Source: CAD feature listing. Evaluate the final solid. Frame: model axes, mm. A direction names the side the tool comes from. Give positions to 0.01 mm unless a question says otherwise; leave off trailing zeros. Order: outer loops, then holes, each group sorted by start corner. A loop starts at its lowest first (then second) coordinate and runs counter-clockwise, first axis right, second up.
from build123d import *

# Parameters (mm, degrees)
SKETCH_1_W           = 15
SKETCH_1_H           = 3
EXTRUDE_1_DEPTH      = 3
SKETCH_2_W           = 15
SKETCH_2_H           = 3
EXTRUDE_2_DEPTH      = 0.5
FILLET_2_R           = 3
FILLET_3_R           = 0.5
FILLET_4_R           = 0.5
SKETCH_6_W           = 103.474287265
SKETCH_6_H           = 3
CUT_EXTRUDE_3_DEPTH  = 10
FILLET_5_R           = 0.5
FILLET_6_R           = 0.5
SKETCH_15_W          = 15
SKETCH_15_H          = 9
EXTRUDE_4_DEPTH      = 3
FILLET_7_R           = 1
SKETCH_16_R          = 1.5
CUT_EXTRUDE_7_DEPTH  = 188.894654659
SKETCH_17_R          = 1.52921897
SKETCH_17_R_2        = 1.502123086
CUT_EXTRUDE_8_DEPTH  = 188.894654659
EXTRUDE_5_DEPTH      = 3
SKETCH_19_R          = 1.5
CUT_EXTRUDE_9_DEPTH  = 10
EXTRUDE_6_DEPTH      = 3
CUT_EXTRUDE_10_DEPTH = 3


with BuildPart() as part:
    # Sketch 1 → Extrude 1 (new body)
    with BuildSketch(Plane.XY):
        Polygon((0, 101), (0, 0), (157.65, 0), (25, 79), (25, 101), (20, 101), (5, 101), align=None)
        with Locations((12.5, 102.5)):
            Rectangle(SKETCH_1_W, SKETCH_1_H)
    extrude(amount=EXTRUDE_1_DEPTH)

    # Sketch 2 → Extrude 2 (add)
    with BuildSketch(Plane(origin=(0, 104, 0), x_dir=(1, 0, 0), z_dir=(0, 1, 0))):
        with Locations((12.5, -1.5)):
            Rectangle(SKETCH_2_W, SKETCH_2_H)
    extrude(amount=EXTRUDE_2_DEPTH)

    # Fillet 2
    fillet_2_edges = [part.edges().sort_by_distance(p)[0] for p in [
        (25, 79, 1.5),
    ]]
    fillet(fillet_2_edges, radius=FILLET_2_R)

    # Fillet 3
    fillet_3_edges = [part.edges().sort_by_distance(p)[0] for p in [
        (157.65, 0, 1.5),
    ]]
    fillet(fillet_3_edges, radius=FILLET_3_R)

    # Fillet 4
    fillet_4_edges = [part.edges().sort_by_distance(p)[0] for p in [
        (0, 0, 1.5),
    ]]
    fillet(fillet_4_edges, radius=FILLET_4_R)

    # Sketch 6 → Cut-Extrude 3 (cut)
    with BuildSketch(Plane.XY.offset(3)):
        with Locations((71.737143632, 1.5)):
            Rectangle(SKETCH_6_W, SKETCH_6_H)
        with BuildLine():
            Line((5, 3), (0, 3))
            Line((0, 3), (0, 0.5))
            ThreePointArc((0, 0.5), (0.146446609, 0.146446609), (0.5, 0))
            Line((0.5, 0), (5, 0))
            Line((5, 0), (5, 3))
        make_face()
        with BuildLine():
            Line((152.612658228, 3), (138.474287265, 3))
            Line((138.474287265, 3), (138.474287265, 0))
            Line((138.474287265, 0), (155.833275758, 0))
            ThreePointArc((155.833275758, 0), (156.315351251, 0.367322877), (156.089117317, 0.929587124))
            Line((156.089117317, 0.929587124), (152.612658228, 3))
        make_face()
    extrude(amount=-CUT_EXTRUDE_3_DEPTH, mode=Mode.SUBTRACT)

    # Fillet 5
    fillet_5_edges = [part.edges().sort_by_distance(p)[0] for p in [
        (123.474287265, 0, 1.5),
        (20, 0, 1.5),
        (138.474287265, 0, 1.5),
        (152.612658228, 3, 1.5),
        (0, 3, 1.5),
        (5, 0, 1.5),
    ]]
    fillet(fillet_5_edges, radius=FILLET_5_R)

    # Fillet 6
    fillet_6_edges = [part.edges().sort_by_distance(p)[0] for p in [
        (123.474287265, 3, 1.5),
        (20, 3, 1.5),
        (5, 101, 1.5),
        (20, 101, 1.5),
        (138.474287265, 3, 1.5),
        (5, 3, 1.5),
    ]]
    fillet(fillet_6_edges, radius=FILLET_6_R)

    # Sketch 15 → Extrude 4 (add)
    with BuildSketch(Plane(origin=(0, 0, 0), x_dir=(-1, 0, 0), z_dir=(0, 0, -1))):
        with Locations((-12.5, 106.877473525)):
            Rectangle(SKETCH_15_W, SKETCH_15_H)
    extrude(amount=-EXTRUDE_4_DEPTH)

    # Fillet 7
    fillet_7_edges = [part.edges().sort_by_distance(p)[0] for p in [
        (5, 111.377473525, 1.5),
        (20, 111.377473525, 1.5),
    ]]
    fillet(fillet_7_edges, radius=FILLET_7_R)

    # Sketch 16 → Cut-Extrude 7 (cut, through all)
    with BuildSketch(Plane(origin=(0, 0, 0), x_dir=(-1, 0, 0), z_dir=(0, 0, -1))):
        with Locations((-14.568919479, 6)):
            Circle(SKETCH_16_R)
        with Locations((-24.568919479, 6)):
            Circle(SKETCH_16_R)
        with Locations((-123.740220593, 6)):
            Circle(SKETCH_16_R)
        with Locations((-133.740220593, 6)):
            Circle(SKETCH_16_R)
    extrude(amount=-CUT_EXTRUDE_7_DEPTH, mode=Mode.SUBTRACT)

    # Sketch 17 → Cut-Extrude 8 (cut, through all)
    with BuildSketch(Plane.XY.offset(3)):
        with Locations((4.795751321, 98)):
            Circle(SKETCH_17_R)
        with Locations((14.795751321, 98)):
            Circle(SKETCH_17_R_2)
    extrude(amount=-CUT_EXTRUDE_8_DEPTH, mode=Mode.SUBTRACT)

    # Sketch 18 → Extrude 5 (add)
    with BuildSketch(Plane.XY.offset(3)):
        with BuildLine():
            Line((19, 130.377473525), (6, 130.377473525))
            ThreePointArc((6, 130.377473525), (5.292893219, 130.084580306), (5, 129.377473525))
            Line((5, 129.377473525), (5, 110.377473525))
            Line((5, 110.377473525), (20, 110.377473525))
            Line((20, 110.377473525), (20, 129.377473525))
            ThreePointArc((20, 129.377473525), (19.707106781, 130.084580306), (19, 130.377473525))
        make_face()
    extrude(amount=-EXTRUDE_5_DEPTH)

    # Sketch 19 → Cut-Extrude 9 (cut)
    with BuildSketch(Plane.XY.offset(3)):
        with Locations((12.5, 127.377473525)):
            Circle(SKETCH_19_R)
        with Locations((12.5, 118.377473525)):
            Circle(SKETCH_19_R)
    extrude(amount=-CUT_EXTRUDE_9_DEPTH, mode=Mode.SUBTRACT)

    # Sketch 21 → Extrude 6 (add)
    with BuildSketch(Plane.XY.offset(3)):
        with BuildLine():
            Line((25, 101), (151.051775545, 3.929587124))
            Line((151.051775545, 3.929587124), (26.464950647, 78.127545412))
            ThreePointArc((26.464950647, 78.127545412), (25.391825537, 79.222696415), (25, 80.705068154))
            Line((25, 80.705068154), (25, 101))
        make_face()
    extrude(amount=-EXTRUDE_6_DEPTH)

    # Sketch 22 → Cut-Extrude 10 (cut)
    with BuildSketch(Plane(origin=(0, 0, 0), x_dir=(-1, 0, 0), z_dir=(0, 0, -1))):
        with BuildLine():
            Line((-19.9, 19), (-19.9, 87.736313508))
            ThreePointArc((-19.9, 87.736313508), (-16, 91.636313508), (-12.1, 87.736313508))
            Line((-12.1, 87.736313508), (-12.1, 19))
            ThreePointArc((-12.1, 19), (-16, 15.1), (-19.9, 19))
        make_face()
        with BuildLine():
            Line((-26.1, 76.955142244), (-26.1, 19))
            ThreePointArc((-26.1, 19), (-30, 15.1), (-33.9, 19))
            Line((-33.9, 19), (-33.9, 76.955142244))
            ThreePointArc((-33.9, 76.955142244), (-30, 80.855142244), (-26.1, 76.955142244))
        make_face()
        with BuildLine():
            Line((-40.1, 66.17397098), (-40.1, 19))
            ThreePointArc((-40.1, 19), (-44, 15.1), (-47.9, 19))
            Line((-47.9, 19), (-47.9, 66.17397098))
            ThreePointArc((-47.9, 66.17397098), (-44, 70.07397098), (-40.1, 66.17397098))
        make_face()
        with BuildLine():
            Line((-54.1, 55.392799717), (-54.1, 19))
            ThreePointArc((-54.1, 19), (-58, 15.1), (-61.9, 19))
            Line((-61.9, 19), (-61.9, 55.392799717))
            ThreePointArc((-61.9, 55.392799717), (-58, 59.292799717), (-54.1, 55.392799717))
        make_face()
        with BuildLine():
            Line((-68.1, 44.611628453), (-68.1, 19))
            ThreePointArc((-68.1, 19), (-72, 15.1), (-75.9, 19))
            Line((-75.9, 19), (-75.9, 44.611628453))
            ThreePointArc((-75.9, 44.611628453), (-72, 48.511628453), (-68.1, 44.611628453))
        make_face()
        with BuildLine():
            Line((-82.1, 33.830457189), (-82.1, 19))
            ThreePointArc((-82.1, 19), (-86, 15.1), (-89.9, 19))
            Line((-89.9, 19), (-89.9, 33.830457189))
            ThreePointArc((-89.9, 33.830457189), (-86, 37.730457189), (-82.1, 33.830457189))
        make_face()
        with BuildLine():
            Line((-96.1, 23.049285925), (-96.1, 19))
            ThreePointArc((-96.1, 19), (-100, 15.1), (-103.9, 19))
            Line((-103.9, 19), (-103.9, 23.049285925))
            ThreePointArc((-103.9, 23.049285925), (-100, 26.949285925), (-96.1, 23.049285925))
        make_face()
    extrude(amount=-CUT_EXTRUDE_10_DEPTH, mode=Mode.SUBTRACT)


solid = part.part
1) First-contact query: pin 1 Ø0.9 at (y, z) = (43, 2) entering from +X; pin 2 Ø1.5 at (y, z) = (27.5, 1) entering from +X; pin 3 Ø0.6 at (y, z) = (1.5, 1.5) entering from -X. Flat tips, straight axial feed; report the tip coordinate or a pass-through.
Checks:
pin 1: stops at x = 100.9
pin 2: stops at x = 121.42
pin 3: stops at x = 5
2) Ray query, L1, parallel to Y at x = 12.5, z = 1.2; L2, parallel to Y at x = 11.5, z = 0.9; L3, parallel to X at y = 40, z = 0.2. Return the intervals inside material, ascending.
Checks:
L1: y = 0 to 17.28, 89.46 to 116.88, 119.88 to 125.88, 128.88 to 130.38
L2: y = 0 to 117.26, 119.5 to 126.26, 128.5 to 130.38
L3: x = 0 to 12.1, 19.9 to 26.1, 33.9 to 40.1, 47.9 to 54.1, 61.9 to 68.1, 75.9 to 104.21
3) Section query A-A on x = 74. Output: boundary loops of the cut face in (y, z).
Checks:
outline: (3, 0) - (15.65, 0) - (15.65, 3) - (3, 3) - close; (47.96, 0) - (63.27, 0) - (63.27, 3) - (47.96, 3) - close
4) Reachability of faces 1 (the face through (53.6, 41.3, 0)), 2 (the face through (47.9, 42, 1)), 3 (the face through (23, 101, 1)), 4 (the face through (2, 101, 1)) from +Z, -Z, +X, -X, +Y, -Y: full face, straight path, thin tool, end or side. Return the list, or none.
Checks:
face 1: -Z, +X, -X, +Y, -Y
face 2: +Z, -Z
face 3: +Z, -Z, +X, +Y
face 4: +Z, -Z, -X, +Y
5) Section query C-C on y = 122. Output: boundary loops of the cut face in (x, z), and give its area (3 significant figures).
Checks:
outline: (5, 0) - (20, 0) - (20, 3) - (5, 3) - close
area: 45.0 mm2
6) Section query B-B on y = 73.5. Output: boundary loops of the cut face in (x, z).
Checks:
outline: (0, 0) - (12.1, 0) - (12.1, 3) - (0, 3) - close; (19.9, 0) - (26.1, 0) - (26.1, 3) - (19.9, 3) - close; (33.9, 0) - (60.71, 0) - (60.71, 3) - (33.9, 3) - close
7) Section query D-D on x = 58. Output: boundary loops of the cut face in (y, z).
Checks:
outline: (3, 0) - (15.1, 0) - (15.1, 3) - (3, 3) - close; (59.29, 0) - (75.59, 0) - (75.59, 3) - (59.29, 3) - close
